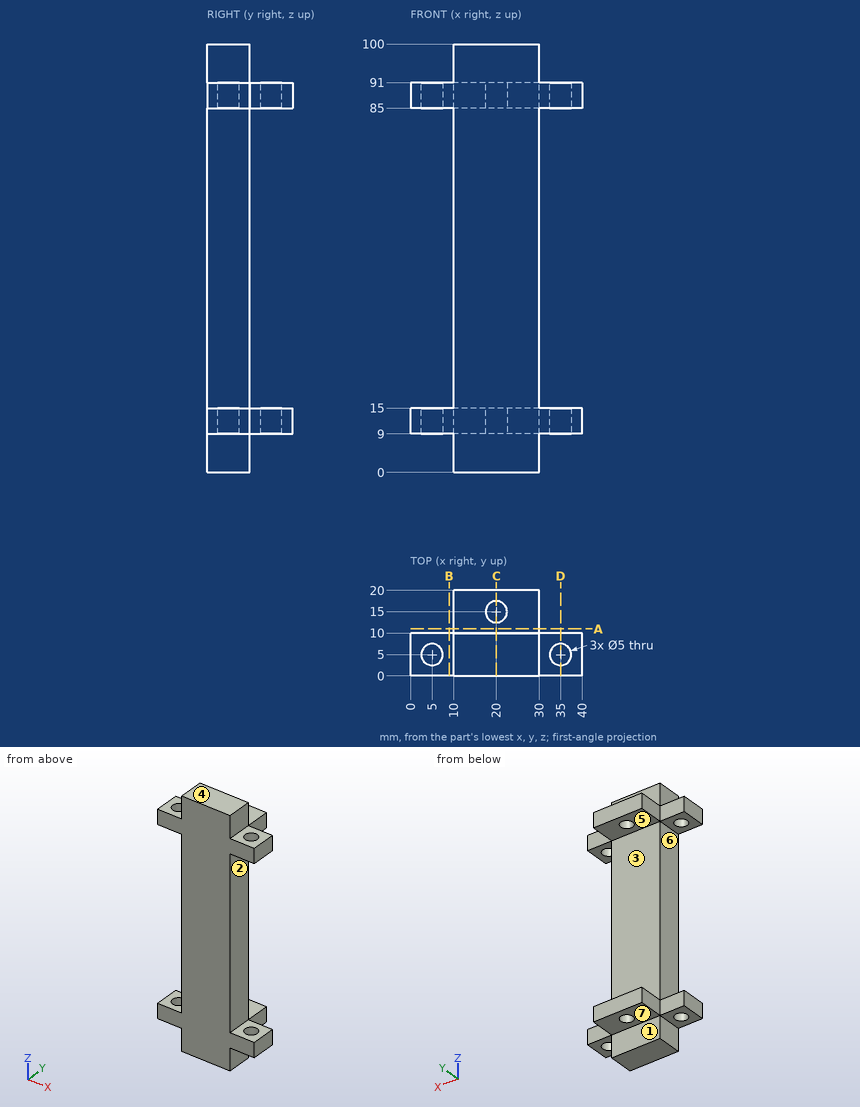
Geometry: see drawing. Coordinates: mm, zero at the bounding-box minimum. A direction names the side the tool comes from. Give positions to 0.01 mm unless a question says otherwise; leave off trailing zeros. Loops run counter-clockwise (first coordinate to the right, second up) from the corner with the lowest first, then second, coordinate; pieces in that order, holes last. Notation, with made-up numbers: (-28, -30) -> (17, -30) arc R21 ccw to (17, -18) -> close; hole circle Ø8 at (-7, -25). An arc over 180 degrees is marked (long way). Use one line per item in the form item = value.
Item 1: Section query B-B on x = 9. Output: boundary loops of the cut face in (y, z).
A:
outline = (0, 9) -> (10, 9) -> (10, 15) -> (0, 15) -> close; (0, 85) -> (10, 85) -> (10, 91) -> (0, 91) -> close
Item 2: Section query D-D on x = 35. Output: boundary loops of the cut face in (y, z).
A:
outline = (0, 9) -> (2.5, 9) -> (2.5, 15) -> (0, 15) -> close; (0, 85) -> (2.5, 85) -> (2.5, 91) -> (0, 91) -> close; (7.5, 9) -> (10, 9) -> (10, 15) -> (7.5, 15) -> close; (7.5, 85) -> (10, 85) -> (10, 91) -> (7.5, 91) -> close
Item 3: Pin query (flat end, axial travel): P1, Ø1.8, axis at y = 13.5, z = 87, coming from the -X side; P2, Ø6, axis at y = 6.5, z = 64.5, coming from the +X side; P3, Ø11, axis at x = 3.5, y = 6, coming from the +Z side. Return the tip coordinate at first contact, or that it passes through.
A:
P1 = 10
P2 = 30
P3 = 91
Item 4: Line query: probe 1 along Y at (x, z) = (20, 12.65); probe 2 along Z at (x, y) = (28, 14.75); probe 3 along Y at (x, z) = (35, 13). Output: solid intervals per line, ascending.
A:
probe_1 = 0 to 12.5, 17.5 to 20
probe_2 = 9 to 15, 85 to 91
probe_3 = 0 to 2.5, 7.5 to 10
Item 5: Section query A-A on y = 11. Output: boundary loops of the cut face in (x, z), and give its area (3 significant figures).
A:
outline = (10, 9) -> (30, 9) -> (30, 15) -> (10, 15) -> close; (10, 85) -> (30, 85) -> (30, 91) -> (10, 91) -> close
area = 240 mm^2
Item 6: Section query C-C on x = 20. Output: boundary loops of the cut face in (y, z).
A:
outline = (0, 0) -> (10, 0) -> (10, 9) -> (12.5, 9) -> (12.5, 15) -> (10, 15) -> (10, 85) -> (12.5, 85) -> (12.5, 91) -> (10, 91) -> (10, 100) -> (0, 100) -> close; (17.5, 9) -> (20, 9) -> (20, 15) -> (17.5, 15) -> close; (17.5, 85) -> (20, 85) -> (20, 91) -> (17.5, 91) -> close
Item 7: Access query for the marked faces 5, 6 and 7. Directions: +Z, -Z, +X, -X, +Y, -Y. A direction counts if a zero-diameter tool reaches every point of the face in a straight line with its end or side. Return the directions, or none.
A:
face_5 = +X, -X, +Y
face_6 = -X, +Y, -Y
face_7 = -Z, +X, -X, +Y
Item 8: Draft query along Z for the marked faces 1, 2, 3 and 4. Return one class per face: pulls with the +Z half, pulls with the -Z half, needs draft (parallel to the pull), parting line crosses it, or undercut.
A:
face_1 = needs draft
face_2 = undercut
face_3 = undercut
face_4 = pulls with the +Z half
